The model under review builds one solid part; all positions refer to its coordinate system, in mm. Give positions to 0.01 mm unless a question says otherwise; leave off trailing zeros. Write each loop counter-clockwise with the first axis right and the second up, starting at its lowest first coordinate (ties: lowest second). Pieces come first, ordered by that corner, then holes. Notation, with made-up numbers: (70.25, 23) - (120.25, 23) arc R19 cw to (120.25, 43) - close; hole circle Ø8 at (88, 5). An arc over 180 degrees is marked (long way). Write item = value, one per line.
```python
from build123d import *

# Parameters (mm, degrees)
F0_R     = 28.8392585449
F1_DEPTH = 6.858
F2_DEPTH = 25.4
F3_R     = 5.08
F4_R     = 5.08


with BuildPart() as f1:
    # F0 (on Front) → F1 (new body)
    with BuildSketch(Plane.XZ):
        Circle(F0_R)
    extrude(amount=F1_DEPTH)

    # F2 (add): a face of the model
    f2_faces = [f1.faces().sort_by_distance(p)[0] for p in [
        (0, -6.858, 0),
    ]]
    extrude(f2_faces, amount=F2_DEPTH)

    # F3
    f3_edges = [f1.edges().sort_by_distance(p)[0] for p in [
        (-28.839259, -32.258, 0),
    ]]
    fillet(f3_edges, radius=F3_R)

    # F4
    f4_edges = [f1.edges().sort_by_distance(p)[0] for p in [
        (28.839259, -13.589, 0),
        (-28.839259, -27.178, 0),
        (-28.839259, 0, 0),
    ]]
    fillet(f4_edges, radius=F4_R)


solid = f1.part
```
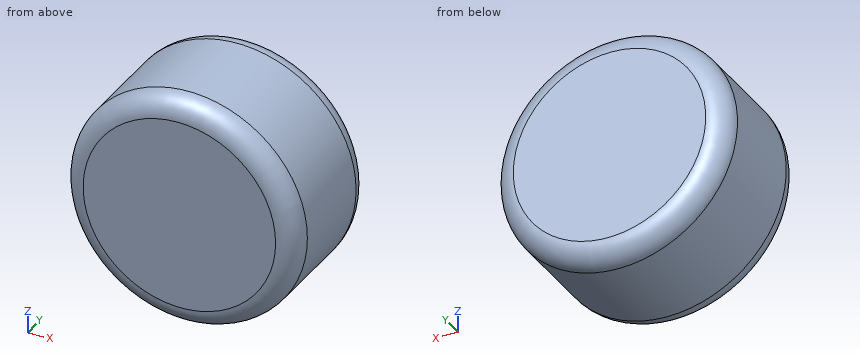
1. Take a section at A-A on y = -13. Give the boundary of the cut face in (x, z), and give its area (3 significant figures).
Findings below:
outline = circle Ø57.68 at (0, 0)
area = 2,610 mm²
2. For line 1 (X direction, y = -9, z = 11); line 2 (Y direction, x = 5, z = 23.5); line 3 (X direction, y = -30, z = 17.5), list the stretches that pass through material, from the lowest coordinate up. Write a range as from..to.
Findings below:
line_1 = -26.66..26.66
line_2 = -32.25..-0.01
line_3 = -21.84..21.84
3. Take a section at B-B on y = -28. Give the boundary of the cut face in (x, z).
Findings below:
outline = circle Ø57.54 at (0, 0)
4. Insertion check: P1, Ø8, axis at y = -26.5, z = -15, coming from the +X side; P2, Ø8, axis at y = -25, z = 18, coming from the +X side; P3, Ø1.5, axis at x = 19, y = -19, coming from the +Z side. Each pin has a flat end and moves straight along its axis. Give the tip position at first contact, or say it passes through.
Findings below:
P1 = 26.66
P2 = 25.21
P3 = 22.33
